Check sheet for the modelled part. Datum: model origin and axes. Units: mm. Face numbers are marked on the shaded views. Coordinates: 2 decimals unless noted, no trailing zeros. Write each loop counter-clockwise with the first axis right and the second up, starting at its lowest first coordinate (ties: lowest second). Pieces come first, ordered by that corner, then holes. Notation, with made-up numbers: M -4,6 L 49,6 A4 cw 49,11 Z; hole C -11.75,12.5 d5. An arc over 180 degrees is marked long. Answer as CSV lines item,"result".
from build123d import *

# Parameters (mm, degrees)
CROQUIS1_R              = 75
SALIENTE_EXTRUIR1_DEPTH = 1600
CROQUIS2_R              = 125
SALIENTE_EXTRUIR2_DEPTH = 50
CROQUIS3_R              = 150
SALIENTE_EXTRUIR3_DEPTH = 50
CROQUIS4_W              = 70
CROQUIS4_H              = 20
CORTAR_EXTRUIR1_DEPTH   = 30


with BuildPart() as part:
    # Croquis1 → Saliente-Extruir1 (new body)
    with BuildSketch(Plane(origin=(0, 0, 0), x_dir=(1, 0, 0), z_dir=(0, 1, 0))):
        with Locations(Location((0, 0, 0), (0, 0, 270))):
            Circle(CROQUIS1_R)
    extrude(amount=SALIENTE_EXTRUIR1_DEPTH)

    # Croquis2 → Saliente-Extruir2 (add)
    with BuildSketch(Plane(origin=(0, 1600, 0), x_dir=(1, 0, 0), z_dir=(0, 1, 0))):
        with Locations(Location((0, 0, 0), (0, 0, 270))):
            Circle(CROQUIS2_R)
    extrude(amount=SALIENTE_EXTRUIR2_DEPTH)

    # Croquis3 → Saliente-Extruir3 (add)
    with BuildSketch(Plane.XZ):
        with Locations(Location((0, 0, 0), (0, 0, 270))):
            Circle(CROQUIS3_R)
    extrude(amount=SALIENTE_EXTRUIR3_DEPTH)

    # Croquis4 → Cortar-Extruir1 (cut)
    with BuildSketch(Plane.XZ.offset(50)):
        with Locations((-65, -5)):
            Rectangle(CROQUIS4_W, CROQUIS4_H)
        with Locations((65, -5)):
            Rectangle(CROQUIS4_W, CROQUIS4_H)
    extrude(amount=-CORTAR_EXTRUIR1_DEPTH, mode=Mode.SUBTRACT)


solid = part.part
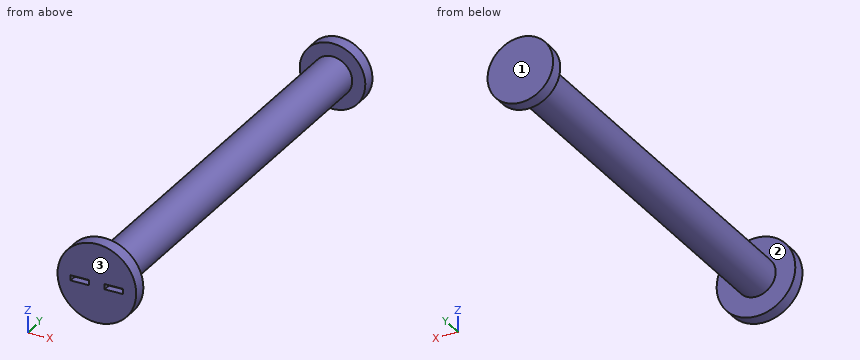
1) Depth check by flat-ended pin: P1, Ø10, axis at x = 65, z = -4.5, coming from the -Y side; P2, Ø15, axis at x = 69, y = -42, coming from the -Z side; P3, Ø1, axis at x = 48.5, y = 924, coming from the +Z side; P4, Ø8, axis at x = -81, y = 796.5, coming from the -Z side. Enter the tip coordinate at first touch or a pass-through.
Answer key:
P1,"stops at y = -20"
P2,"stops at z = -136.81"
P3,"stops at z = 57.63"
P4,"passes through"
2) Mould release check, pull along Y, two halves, no side actions. Record for the marked faces 1, 2 and 3: pulls with the +Y half, pulls with the -Y half, needs draft (parallel to the pull), parting line crosses it, or undercut.
Answer key:
face 1,"pulls with the +Y half"
face 2,"undercut"
face 3,"pulls with the -Y half"
3) Section check A-A, the plane z = 97. Record the boundary of the cut face in (x, y), plus the area to 3 significant figures.
Answer key:
outline,"M -114.42,-50 L 114.42,-50 L 114.42,0 L -114.42,0 Z; M -78.84,1600 L 78.84,1600 L 78.84,1650 L -78.84,1650 Z"
area,"19,300 mm2"
4) Section check C-C, the plane y = 1374. Record the boundary of the cut face in (x, z), plus the area to 3 significant figures.
Answer key:
outline,"C 0,0 d150"
area,"17,700 mm2"
5) Section check B-B, the plane x = 0. Record the boundary of the cut face in (y, z), plus the area to 4 significant figures.
Answer key:
outline,"M -50,-150 L 0,-150 L 0,-75 L 1600,-75 L 1600,-125 L 1650,-125 L 1650,125 L 1600,125 L 1600,75 L 0,75 L 0,150 L -50,150 Z"
area,"267,500 mm2"
6) Thickness scan on line 1 along Y through (x, z) = (-76, -67); line 2 along X through (y, z) = (607, -2.5); line 3 along Y through (x, z) = (117.5, -86). Record the ranges inside material, lowest first.
Answer key:
line 1,"y = -50 to 0, 1600 to 1650"
line 2,"x = -74.96 to 74.96"
line 3,"y = -50 to 0"
